Here's how the part is built. I have some questions about the finished solid (model axes, mm). Face numbers are marked on the shaded views. Give positions to 0.01 mm unless a question says otherwise; leave off trailing zeros. Loops run counter-clockwise (first coordinate to the right, second up) from the corner with the lowest first, then second, coordinate; pieces in that order, holes last.
Q1. If we section it at D-D (z = -18): Please give me the cut outline in (x, y) (3 decimals).
Q2. If we section it at B-B (x = 16): Please give me the cut outline in (y, z), plus the area to 3 significant figures.
Q3. Will these pins go through, and if not, where does the flat tip stop? P1, Ø2.5, axis at x = -36.5, z = -53, coming from the -Y side; P2, Ø1.5, axis at x = 4.5, z = 7, coming from the +Y side; P3, Ø1, axis at x = 8.5, y = -1, coming from the +Z side.
Q4. If we section it at C-C (y = 13.5): Please give me the cut outline in (x, z) (3 decimals), plus the area to 3 significant figures.
Q5. I need wall thicknesses on line 1 (Z direction, x = -21, y = 13.5); line 2 (X direction, y = 13.25, z = 19) (3 decimals); line 3 (Z direction, x = 1, y = -3). Which ranges of each line are inside material? Lowest first, please.
Q6. If we section it at A-A (y = 6.25): Please give me the cut outline in (x, z) (3 decimals).
Q7. We'd pull the mould along X, two halves only. Please class the marked faces 1, 2 and 3: +X half, -X half, draft (parallel to the pull), parting line (faces both ways), or undercut.
from build123d import *

# Parameters (mm, degrees)
SKETCH1_W           = 75.85
SKETCH1_H           = 158.4
BOSS_EXTRUDE1_DEPTH = 3
SKETCH2_W           = 75.85
SKETCH2_H           = 158.4
SKETCH2_W_2         = 69.85
SKETCH2_H_2         = 152.4
BOSS_EXTRUDE2_DEPTH = 17.78
SKETCH3_W           = 12.7
SKETCH3_H           = 8.89
BOSS_EXTRUDE3_DEPTH = 3.81
CUT_EXTRUDE4_REACH  = 92.237
SKETCH4_R           = 1.7
SKETCH4_R_2         = 1.72
CUT_EXTRUDE5_REACH  = 166.197
SKETCH10_W          = 58.42
SKETCH10_H          = 8.89
CUT_EXTRUDE6_REACH  = 113.614
SKETCH11_W          = 30.48
SKETCH11_H          = 7.62
SKETCH12_W          = 17.78
SKETCH12_H          = 5.08
BOSS_EXTRUDE4_DEPTH = 5.08
SKETCH13_W          = 17.78
SKETCH13_H          = 2.54
BOSS_EXTRUDE5_DEPTH = 5.08


with BuildPart() as part:
    # Sketch1 → Boss-Extrude1 (new body)
    with BuildSketch(Plane(origin=(0, 0, 0), x_dir=(1, 0, 0), z_dir=(0, 1, 0))):
        Rectangle(SKETCH1_W, SKETCH1_H)
    extrude(amount=BOSS_EXTRUDE1_DEPTH)

    # Sketch2 → Boss-Extrude2 (add)
    with BuildSketch(Plane(origin=(0, 3, 0), x_dir=(1, 0, 0), z_dir=(0, 1, 0))):
        Rectangle(SKETCH2_W, SKETCH2_H)
        Rectangle(SKETCH2_W_2, SKETCH2_H_2, mode=Mode.SUBTRACT)
    extrude(amount=BOSS_EXTRUDE2_DEPTH)

    # Sketch3 → Boss-Extrude3 (add)
    with BuildSketch(Plane(origin=(0, 20.78, 0), x_dir=(1, 0, 0), z_dir=(0, 1, 0))):
        with Locations((-28.575, 71.755)):
            Rectangle(SKETCH3_W, SKETCH3_H)
        with Locations((-28.575, -71.755)):
            Rectangle(SKETCH3_W, SKETCH3_H)
        with Locations((28.575, 71.755)):
            Rectangle(SKETCH3_W, SKETCH3_H)
        with Locations((28.575, -71.755)):
            Rectangle(SKETCH3_W, SKETCH3_H)
    extrude(amount=-BOSS_EXTRUDE3_DEPTH)

    # Sketch4 → Cut-Extrude4 (cut, up to next)
    with BuildSketch(Plane(origin=(0, 20.78, 0), x_dir=(1, 0, 0), z_dir=(0, 1, 0)), mode=Mode.PRIVATE) as cut_extrude4_sk1:
        with Locations(Location((-28.575, 73.025, 0), (0, 0, 270))):
            Circle(SKETCH4_R)
    cut_extrude4_tool1 = extrude(cut_extrude4_sk1.sketch, amount=-CUT_EXTRUDE4_REACH, mode=Mode.PRIVATE) & part.part
    # Sketch4 → Cut-Extrude4 (cut, up to next)
    with BuildSketch(Plane(origin=(0, 20.78, 0), x_dir=(1, 0, 0), z_dir=(0, 1, 0)), mode=Mode.PRIVATE) as cut_extrude4_sk2:
        with Locations(Location((28.575, 73.025, 0), (0, 0, 270))):
            Circle(SKETCH4_R)
    cut_extrude4_tool2 = extrude(cut_extrude4_sk2.sketch, amount=-CUT_EXTRUDE4_REACH, mode=Mode.PRIVATE) & part.part
    # Sketch4 → Cut-Extrude4 (cut, up to next)
    with BuildSketch(Plane(origin=(0, 20.78, 0), x_dir=(1, 0, 0), z_dir=(0, 1, 0)), mode=Mode.PRIVATE) as cut_extrude4_sk3:
        with Locations(Location((28.575, -73.025, 0), (0, 0, 270))):
            Circle(SKETCH4_R_2)
    cut_extrude4_tool3 = extrude(cut_extrude4_sk3.sketch, amount=-CUT_EXTRUDE4_REACH, mode=Mode.PRIVATE) & part.part
    # Sketch4 → Cut-Extrude4 (cut, up to next)
    with BuildSketch(Plane(origin=(0, 20.78, 0), x_dir=(1, 0, 0), z_dir=(0, 1, 0)), mode=Mode.PRIVATE) as cut_extrude4_sk4:
        with Locations(Location((-28.575, -73.025, 0), (0, 0, 270))):
            Circle(SKETCH4_R)
    cut_extrude4_tool4 = extrude(cut_extrude4_sk4.sketch, amount=-CUT_EXTRUDE4_REACH, mode=Mode.PRIVATE) & part.part
    add(cut_extrude4_tool1.solids().sort_by_distance((-28.575, 20.78, -73.025))[0], mode=Mode.SUBTRACT)
    add(cut_extrude4_tool2.solids().sort_by_distance((28.575, 20.78, -73.025))[0], mode=Mode.SUBTRACT)
    add(cut_extrude4_tool3.solids().sort_by_distance((28.575, 20.78, 73.025))[0], mode=Mode.SUBTRACT)
    add(cut_extrude4_tool4.solids().sort_by_distance((-28.575, 20.78, 73.025))[0], mode=Mode.SUBTRACT)

    # Sketch10 → Cut-Extrude5 (cut, up to next)
    with BuildSketch(Plane(origin=(0, 0, -79.2), x_dir=(-1, 0, 0), z_dir=(0, 0, -1)), mode=Mode.PRIVATE) as cut_extrude5_sk1:
        with Locations((0, 7.445)):
            Rectangle(SKETCH10_W, SKETCH10_H)
    cut_extrude5_tool1 = extrude(cut_extrude5_sk1.sketch, amount=-CUT_EXTRUDE5_REACH, mode=Mode.PRIVATE) & part.part
    add(cut_extrude5_tool1.solids().sort_by_distance((0, 7.445, -79.2))[0], mode=Mode.SUBTRACT)

    # Sketch11 → Cut-Extrude6 (cut, up to next)
    with BuildSketch(Plane.ZY.offset(37.925), mode=Mode.PRIVATE) as cut_extrude6_sk1:
        with Locations((-56.34, 6.858)):
            Rectangle(SKETCH11_W, SKETCH11_H)
    cut_extrude6_tool1 = extrude(cut_extrude6_sk1.sketch, amount=-CUT_EXTRUDE6_REACH, mode=Mode.PRIVATE) & part.part
    add(cut_extrude6_tool1.solids().sort_by_distance((-37.925, 6.858, -56.34))[0], mode=Mode.SUBTRACT)

    # Sketch12 → Boss-Extrude4 (add)
    with BuildSketch(Plane.XZ):
        with Locations((0, 12.7)):
            Rectangle(SKETCH12_W, SKETCH12_H)
        with Locations((0, -12.7)):
            Rectangle(SKETCH12_W, SKETCH12_H)
    extrude(amount=BOSS_EXTRUDE4_DEPTH)

    # Sketch13 → Boss-Extrude5 (add)
    with BuildSketch(Plane(origin=(0, 0, 10.16), x_dir=(-1, 0, 0), z_dir=(0, 0, -1))):
        with Locations((0, -3.81)):
            Rectangle(SKETCH13_W, SKETCH13_H)
    boss_extrude5 = extrude(amount=BOSS_EXTRUDE5_DEPTH)

    # Mirror1: Boss-Extrude5 across plane
    add(boss_extrude5.mirror(Plane(origin=(0, 0, 0), x_dir=(1, 0, 0), z_dir=(0, 0, -1))))


solid = part.part
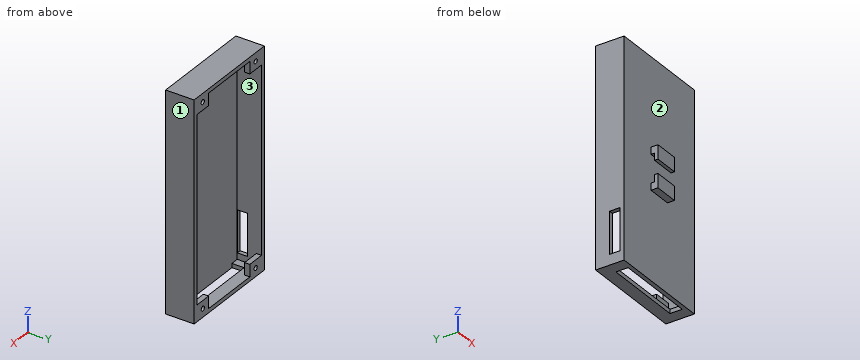
Check sheet entries:
1. outline: (-37.925, 0) - (37.925, 0) - (37.925, 20.78) - (34.925, 20.78) - (34.925, 3) - (-34.925, 3) - (-34.925, 20.78) - (-37.925, 20.78) - close
2. outline: (0, -79.2) - (3, -79.2) - (3, 76.2) - (20.78, 76.2) - (20.78, 79.2) - (0, 79.2) - close; (11.89, -79.2) - (20.78, -79.2) - (20.78, -76.2) - (11.89, -76.2) - close
2. area: 555 mm2
3. P1: stops at y = 0
3. P2: stops at y = 3
3. P3: stops at z = 15.24
4. outline: (-37.925, -79.2) - (37.925, -79.2) - (37.925, 79.2) - (-37.925, 79.2) - close; hole (-34.925, -76.2) - (34.925, -76.2) - (34.925, 76.2) - (-34.925, 76.2) - close
4. area: 1,370 mm2
5. line 1: z = -79.2 to -76.2, 76.2 to 79.2
5. line 2: x = -37.925 to -34.925, 34.925 to 37.925
5. line 3: z = -15.24 to -5.08, 5.08 to 15.24
6. outline: (-37.925, -79.2) - (-29.21, -79.2) - (-29.21, -76.2) - (-34.925, -76.2) - (-34.925, -71.58) - (-37.925, -71.58) - close; (-37.925, -41.1) - (-34.925, -41.1) - (-34.925, 76.2) - (34.925, 76.2) - (34.925, -76.2) - (29.21, -76.2) - (29.21, -79.2) - (37.925, -79.2) - (37.925, 79.2) - (-37.925, 79.2) - close
7. face 1: +X half
7. face 2: draft
7. face 3: undercut
